from build123d import *

# Parameters (mm, degrees)
F0_W     = 304.8
F0_H     = 152.4
F1_DEPTH = 5.207
F2_W     = 177.8
F2_H     = 114.3
F3_DEPTH = 5.208
F4_R     = 19.05
F5_DEPTH = 5.208
F6_R     = 11.1125
F7_DEPTH = 5.208
F10_R    = 5.08
F11_R    = 5.08


with BuildPart() as f1:
    # F0 (on Top) → F1 (new body)
    with BuildSketch(Plane.XY):
        Rectangle(F0_W, F0_H)
    extrude(amount=F1_DEPTH)

    # F2 (on face) → F3 (cut, through all)
    with BuildSketch(Plane.XY.offset(5.207)):
        Rectangle(F2_W, F2_H)
    extrude(amount=-F3_DEPTH, mode=Mode.SUBTRACT)

    # F4 (on face) → F5 (cut, through all)
    with BuildSketch(Plane.XY.offset(5.207)):
        with Locations((120.65, -44.45)):
            Circle(F4_R)
        with Locations((120.65, 0)):
            Circle(F4_R)
        with Locations((120.65, 44.45)):
            Circle(F4_R)
    extrude(amount=-F5_DEPTH, mode=Mode.SUBTRACT)

    # F6 (on face) → F7 (cut, through all)
    with BuildSketch(Plane.XY.offset(5.207)):
        with Locations((-134.9375, 52.3875)):
            Circle(F6_R)
        with Locations((-106.3625, 52.3875)):
            Circle(F6_R)
        with Locations((-134.9375, 17.7927)):
            Circle(F6_R)
        with Locations((-106.3625, 17.7927)):
            Circle(F6_R)
        with Locations((-134.9375, -17.4625)):
            Circle(F6_R)
        with Locations((-106.3625, -17.4625)):
            Circle(F6_R)
        with Locations((-134.9375, -52.3875)):
            Circle(F6_R)
        with Locations((-106.3625, -52.3875)):
            Circle(F6_R)
    extrude(amount=-F7_DEPTH, mode=Mode.SUBTRACT)

    # F10
    f10_edges = [f1.edges().sort_by_distance(p)[0] for p in [
        (-152.4, -76.2, 2.6035),
        (-152.4, 76.2, 2.6035),
        (152.4, 76.2, 2.6035),
        (152.4, -76.2, 2.6035),
    ]]
    fillet(f10_edges, radius=F10_R)

    # F11
    f11_edges = [f1.edges().sort_by_distance(p)[0] for p in [
        (-88.9, 57.15, 2.6035),
        (-88.9, -57.15, 2.6035),
        (88.9, 57.15, 2.6035),
        (88.9, -57.15, 2.6035),
    ]]
    fillet(f11_edges, radius=F11_R)


with BuildPart() as f8_1:
    # F8: copy of F1
    add(f1.part)


solid = f1.part
The model under review builds one solid part; all positions refer to its coordinate system, in mm. A direction names the side the tool comes from. Give positions to 0.01 mm unless a question says otherwise; leave off trailing zeros. Write each loop counter-clockwise with the first axis right and the second up, starting at its lowest first coordinate (ties: lowest second). Pieces come first, ordered by that corner, then holes.
1. Add section C-C, the plane x = 61. Write out the cut boundary in (y, z).
2. Add section B-B, the plane x = 120.65. Write out the cut boundary in (y, z), plus the area to 3 significant figures.
3. Draft analysis for pull direction Y (two halves, no side actions). For faces 3 (the cylindrical face through (-95.763, 55.725, 2.64)), 4 (the flat face through (-2, -76.2, 3)), 5 (the flat face through (-2, -67, 5.207)), state which applies: +Y half, -Y half, draft (parallel to the pull), parting line (faces both ways), or undercut.
4. Add section A-A, the plane y = 0. Write out the cut boundary in (x, z), plus the area to 3 significant figures.
5. Wall thickness on L1, parallel to Y at x = 120.65, z = 4; L2, parallel to Y at x = -70, z = 2.4; L3, parallel to X at y = -12.5, z = 2.7: over which ranges is each line inside the solid? List them lowest first.
6. For P1, Ø23, axis at x = 120.65, y = 44.45, coming from the +Z side, flat-tipped, find the tip position at first contact; note if it passes through.
7. Tool access review of faces 1 (the flat face through (-1, -57.15, 3)), 2 (the flat face through (152.4, -1, 3)): name each direction out of +Z, -Z, +X, -X, +Y, -Y from which nothing blocks a thin tool from reaching the whole face with its end or side.
8. Add section D-D, the plane z = 1.9. Count the separate pieces of the cut face and the enclosed holes in it, plus the area to 3 significant figures.
Worked answers:
1. outline: (-76.2, 0) - (-57.15, 0) - (-57.15, 5.21) - (-76.2, 5.21) - close; (57.15, 0) - (76.2, 0) - (76.2, 5.21) - (57.15, 5.21) - close
2. outline: (-76.2, 0) - (-63.5, 0) - (-63.5, 5.21) - (-76.2, 5.21) - close; (-25.4, 0) - (-19.05, 0) - (-19.05, 5.21) - (-25.4, 5.21) - close; (19.05, 0) - (25.4, 0) - (25.4, 5.21) - (19.05, 5.21) - close; (63.5, 0) - (76.2, 0) - (76.2, 5.21) - (63.5, 5.21) - close
2. area: 198 mm2
3. face 3: undercut
3. face 4: -Y half
3. face 5: draft
4. outline: (-152.4, 0) - (-88.9, 0) - (-88.9, 5.21) - (-152.4, 5.21) - close; (88.9, 0) - (101.6, 0) - (101.6, 5.21) - (88.9, 5.21) - close; (139.7, 0) - (152.4, 0) - (152.4, 5.21) - (139.7, 5.21) - close
4. area: 463 mm2
5. L1: y = -76.2 to -63.5, -25.4 to -19.05, 19.05 to 25.4, 63.5 to 76.2
5. L2: y = -76.2 to -57.15, 57.15 to 76.2
5. L3: x = -152.4 to -144.88, -124.99 to -116.31, -96.42 to -88.9, 88.9 to 106.27, 135.03 to 152.4
6. P1: passes through
7. face 1: +Z, -Z
7. face 2: +Z, -Z, +X, +Y, -Y
8. separate pieces: 1
8. enclosed holes: 12
8. area: 19,600 mm2
